Verification items for the finished model (mm, model axes). Face numbers are marked on the shaded views. Round coordinates to 2 decimals unless told otherwise and drop trailing zeros. Loops run counter-clockwise (first coordinate to the right, second up) from the corner with the lowest first, then second, coordinate; pieces in that order, holes last. Notation, with made-up numbers: (-18.75, -2.5) - (7.25, -2.5) arc R14 ccw to (7.25, 19.5) - close; hole circle Ø6 at (-6.5, 65). An arc over 180 degrees is marked (long way). Use CSV: the item, a comma, the result in double quotes.
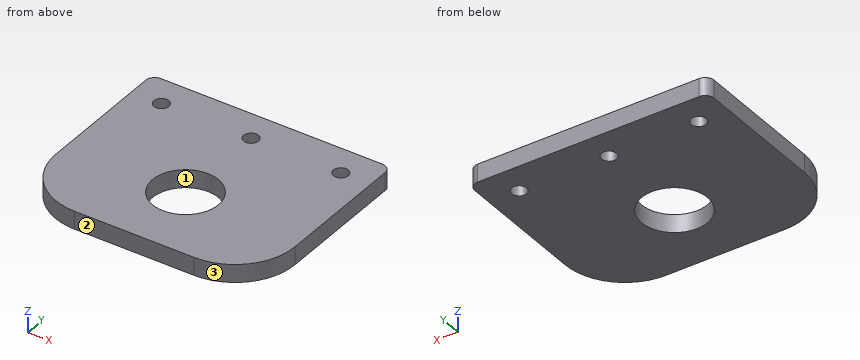
```python
from build123d import *

# Parameters (mm, degrees)
SKETCH_1_W          = 80
SKETCH_1_H          = 67
SKETCH_1_R          = 11
EXTRUDE_1_DEPTH     = 6
SKETCH_2_R          = 2.5
CUT_EXTRUDE_1_DEPTH = 10
FILLET_1_R          = 20
FILLET_2_R          = 3


with BuildPart() as part:
    # 草图1 → 凸台-拉伸1 (new body)
    with BuildSketch(Plane.XY):
        Rectangle(SKETCH_1_W, SKETCH_1_H)
        with Locations((0, -8.5)):
            Circle(SKETCH_1_R, mode=Mode.SUBTRACT)
    extrude(amount=EXTRUDE_1_DEPTH)

    # 草图2 → 切除-拉伸1 (cut)
    with BuildSketch(Plane(origin=(0, 0, 0), x_dir=(-1, 0, 0), z_dir=(0, 0, -1))):
        with Locations((-30, 23.5)):
            Circle(SKETCH_2_R)
        with Locations((30, 23.5)):
            Circle(SKETCH_2_R)
        with Locations((0, 23.5)):
            Circle(SKETCH_2_R)
    extrude(amount=-CUT_EXTRUDE_1_DEPTH, mode=Mode.SUBTRACT)

    # 圆角1
    fillet_1_edges = [part.edges().sort_by_distance(p)[0] for p in [
        (40, -33.5, 3),
        (-40, -33.5, 3),
    ]]
    fillet(fillet_1_edges, radius=FILLET_1_R)

    # 圆角2
    fillet_2_edges = [part.edges().sort_by_distance(p)[0] for p in [
        (-40, 33.5, 3),
        (40, 33.5, 3),
    ]]
    fillet(fillet_2_edges, radius=FILLET_2_R)


solid = part.part
```
1) Cross-section at D-D, the plane x = -30. Record the cut outline in (y, z), then the cut area to 3 significant figures.
Returned:
outline,"(-30.82, 0) - (21, 0) - (21, 6) - (-30.82, 6) - close; (26, 0) - (33.5, 0) - (33.5, 6) - (26, 6) - close"
area,"356 mm²"
2) Gauge pin test, flat ends, axial feed: pin 1 Ø1 at (x, y) = (-29, 4.5) entering from -Z; pin 2 Ø3 at (x, y) = (30, 23.5) entering from -Z; pin 3 Ø3 at (y, z) = (-19.5, 0.5) entering from -X. Record the tip position at first contact, or that the pin passes through.
Returned:
pin 1,"stops at z = 0"
pin 2,"passes through"
pin 3,"stops at x = -39.49"
3) Cross-section at B-B, the plane y = 25. Record the cut outline in (x, z).
Returned:
outline,"(-40, 0) - (-32, 0) - (-32, 6) - (-40, 6) - close; (-28, 0) - (-2, 0) - (-2, 6) - (-28, 6) - close; (2, 0) - (28, 0) - (28, 6) - (2, 6) - close; (32, 0) - (40, 0) - (40, 6) - (32, 6) - close"
4) Cross-section at A-A, the plane x = 0. Record the cut outline in (y, z).
Returned:
outline,"(-33.5, 0) - (-19.5, 0) - (-19.5, 6) - (-33.5, 6) - close; (2.5, 0) - (21, 0) - (21, 6) - (2.5, 6) - close; (26, 0) - (33.5, 0) - (33.5, 6) - (26, 6) - close"
5) Cross-section at C-C, the plane y = -8.5. Record the cut outline in (x, z).
Returned:
outline,"(-40, 0) - (-11, 0) - (-11, 6) - (-40, 6) - close; (11, 0) - (40, 0) - (40, 6) - (11, 6) - close"
6) Mould release check, pull along X, two halves, no side actions. Record for the marked faces 1, 2 and 3: +X half, -X half, draft (parallel to the pull), parting line (faces both ways), or undercut.
Returned:
face 1,"undercut"
face 2,"draft"
face 3,"+X half"
7) Thickness scan on probe 1 along Y at (x, z) = (-2, 2.55); probe 2 along Y at (x, z) = (0, 3.35); probe 3 along X at (y, z) = (22.5, 4.55). Record the ranges inside material, lowest first. Write a range as [from, to].
Returned:
probe 1,"y = [-33.5, -19.32], [2.32, 22], [25, 33.5]"
probe 2,"y = [-33.5, -19.5], [2.5, 21], [26, 33.5]"
probe 3,"x = [-40, -32.29], [-27.71, -2.29], [2.29, 27.71], [32.29, 40]"
